from build123d import *
from build123d import SkipClean  # not in build123d's __all__

# Parameters (mm, degrees)
F0_R     = 1.5
F1_DEPTH = 15
F3_W     = 10
F3_H     = 4
F5_DEPTH = 45.85
F6_DEPTH = 10
F7_R     = 1.6
F8_DEPTH = 14.001


# Not quite as in the source:
# - after a boolean that leaves OpenCascade's solid faulty, fix() repairs it


with BuildPart() as f1:
    # F0 (on Top) → F1 (new body)
    with BuildSketch(Plane.XY):
        with BuildLine():
            ThreePointArc((9.1651513899, -4), (9.7890631293, -2.0430964369), (10, 0))
            ThreePointArc((10, 0), (9.7890631293, 2.0430964369), (9.1651513899, 4))
            Line((9.1651513899, 4), (-9.1651513899, 4))
            ThreePointArc((-9.1651513899, 4), (-10, 0), (-9.1651513899, -4))
            Line((-9.1651513899, -4), (9.1651513899, -4))
        make_face()
        Circle(F0_R, mode=Mode.SUBTRACT)
        with BuildLine():
            ThreePointArc((-9.1651513899, -4), (0, -10), (9.1651513899, -4))
            Line((9.1651513899, -4), (-9.1651513899, -4))
        make_face()
        with BuildLine():
            Line((-9.1651513899, 4), (9.1651513899, 4))
            ThreePointArc((9.1651513899, 4), (0, 10), (-9.1651513899, 4))
        make_face()
    extrude(amount=-F1_DEPTH)

    # F3 (on offset) → F5 (cut, through all)
    with BuildSketch(Plane.XZ.offset(40)):
        with Locations((0, -10)):
            Rectangle(F3_W, F3_H)
    extrude(amount=-F5_DEPTH, mode=Mode.SUBTRACT)

    # F0 (on Top) → F6 (join)
    with BuildSketch(Plane.XY):
        with BuildLine():
            ThreePointArc((9.1651513899, -4), (9.7890631293, -2.0430964369), (10, 0))
            ThreePointArc((10, 0), (9.7890631293, 2.0430964369), (9.1651513899, 4))
            Line((9.1651513899, 4), (-9.1651513899, 4))
            ThreePointArc((-9.1651513899, 4), (-10, 0), (-9.1651513899, -4))
            Line((-9.1651513899, -4), (9.1651513899, -4))
        make_face()
        Circle(F0_R, mode=Mode.SUBTRACT)
        Circle(F0_R)
    with SkipClean():  # cleaning this boolean's faces spoils the solid; the shape is the same uncleaned
        extrude(amount=F6_DEPTH)

    # F7 (on face) → F8 (cut, through all)
    with BuildSketch(Plane.XZ.offset(4)):
        with Locations((-3, 3.6)):
            Circle(F7_R)
        with Locations((3, 3.6)):
            Circle(F7_R)
    extrude(amount=-F8_DEPTH, mode=Mode.SUBTRACT)

    add(f1.part.fix(), mode=Mode.REPLACE)


solid = f1.part
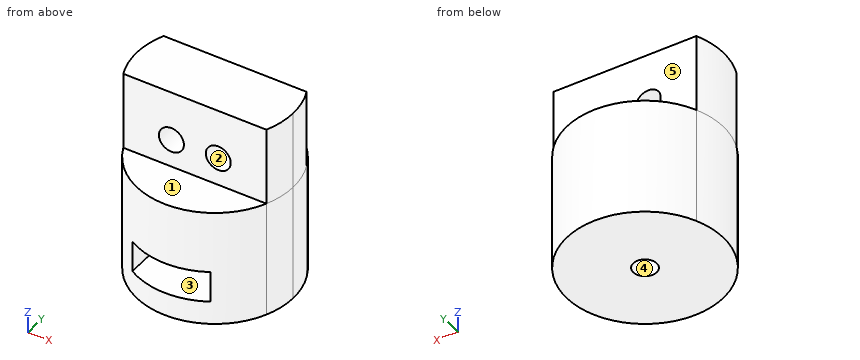
Input: part model. Units: mm. Frame: model coordinates. Face numbers are marked on the shaded views. A direction names the side the tool comes from. Give positions to 0.01 mm unless a question says otherwise; leave off trailing zeros. Loops run counter-clockwise (first coordinate to the right, second up) from the corner with the lowest first, then second, coordinate; pieces in that order, holes last. Notation, with made-up numbers: (-16, 89.25) -> (35, 89.25) arc R27 cw to (35, 115.25) -> close; hole circle Ø6 at (11, -7). An arc over 180 degrees is marked (long way). Answer as a JSON object with one key per item and string values. Group by question number.
Item 1: Cut plane B-B, the plane x = 0. Return the cut outline in (y, z), and give its area (3 significant figures).
Item 2: Pin query (flat end, axial travel): P1, Ø8, axis at x = 3.5, z = 7, coming from the -Y side; P2, Ø12, axis at y = 6.5, z = -1, coming from the +X side; P3, Ø2, axis at x = 6.5, z = -8, coming from the +Y side. Return the tip coordinate at first contact, or that it passes through.
Item 3: Cut plane D-D, the plane z = -8.5. Return the cut outline in (x, y), and give its area (3 significant figures).
Item 4: Pull-direction query (X, two-part tool) for the marked faces 1 and 2; classes: released by +X, released by -X, zero draft, split by the parting line, or undercut.
Item 5: Reachability of the marked faces 3, 4 and 5 from +Z, -Z, +X, -X, +Y, -Y: full face, straight path, thin tool, end or side. Return the list, or none.
Item 6: Cut plane A-A, the plane z = 3.6. Return the cut outline in (x, y).
Item 7: Line query: probe 1 along Y at (x, z) = (0, -12.7); probe 2 along Z at (x, y) = (-4.75, -2.5); probe 3 along Z at (x, y) = (-2.25, -8). Output: solid intervals per line, ascending.
Item 8: Cut plane C-C, the plane z = -2. Return the cut outline in (x, y), and give its area (3 significant figures).
Checks:
{
 "1": {"outline": "(-10, -15) -> (-1.5, -15) -> (-1.5, -12) -> (-10, -12) -> close; (-10, -8) -> (-1.5, -8) -> (-1.5, 0) -> (1.5, 0) -> (1.5, -8) -> (5.85, -8) -> (5.85, -12) -> (1.5, -12) -> (1.5, -15) -> (10, -15) -> (10, 0) -> (4, 0) -> (4, 10) -> (-4, 10) -> (-4, 0) -> (-10, 0) -> close", "area": "284 mm²"},
 "2": {"P1": "stops at y = -4", "P2": "stops at x = 9.99", "P3": "stops at y = 8.35"},
 "3": {"outline": "(-5, -8.66) -> (-5, 5.85) -> (5, 5.85) -> (5, -8.66) arc R10 ccw (long way) to start", "area": "160 mm²"},
 "4": {"face 1": "zero draft", "face 2": "undercut"},
 "5": {"face 3": "-Y", "face 4": "-Z", "face 5": "+Z, +X, -X, +Y"},
 "6": {"outline": "(-9.17, -4) -> (-4.6, -4) -> (-4.6, 4) -> (-9.17, 4) arc R10 ccw to start; (-1.4, -4) -> (1.4, -4) -> (1.4, 4) -> (-1.4, 4) -> close; (4.6, -4) -> (9.17, -4) arc R10 ccw to (9.17, 4) -> (4.6, 4) -> close"},
 "7": {"probe 1": "y = -10 to -1.5, 1.5 to 10", "probe 2": "z = -15 to -12, -8 to 10", "probe 3": "z = -15 to -12, -8 to 0"},
 "8": {"outline": "circle Ø20 at (0, 0); hole circle Ø3 at (0, 0)", "area": "307 mm²"}
}
